Design review of the part built by this model. Coordinates are the model's own, in mm. A direction names the side the tool comes from. Round coordinates to 2 decimals unless told otherwise and drop trailing zeros. Order: outer loops, then holes, each group sorted by start corner. A loop starts at its lowest first (then second) coordinate and runs counter-clockwise, first axis right, second up. Notation, with made-up numbers: M -13,41 L 21,41 A19 cw 21,72 Z; hole C -15.75,85.25 d11. An arc over 180 degrees is marked long. Write each question's results on one line, items separated by ' | '. Start each with the question number.
Item 1: Wall thickness on line 1 (Y direction, x = 37, z = -0.35); line 2 (X direction, y = -19.05, z = -9); line 3 (Y direction, x = 8, z = -10.75): over which ranges is each line inside the solid? List them lowest first. Write a range as [from, to].
Item 2: Machinability: for faces 1 (the flat face through (-28, 0, -2)), 2 (the flat face through (12, 20, -11)), 3 (the cylindrical face through (-9.93, -20.09, -9.88)), which of the approach directions +Z, -Z, +X, -X, +Y, -Y give a long, thin tool a straight path to every point of the face, cutting with its end or side? Answer none if there is none.
Item 3: Take a section at A-A, the plane y = 0. Write out the cut boundary in (x, z), plus the area to 3 significant figures.
Item 4: Take a section at B-B, the plane x = 0. Write out the cut boundary in (y, z).
Item 5: Take a section at D-D, the plane z = -9. Write out the cut boundary in (x, y).
Item 6: Clearance check with flat-ended pins moving along their axes: pin 1 (9.5 mm diameter, centred on x = 40, y = 17.5, fed in from -Z); pin 2 (5 mm diameter, centred on y = -20.5, z = -14, fed in from +X); pin 3 (18 mm diameter, centred on x = -37, y = 0, fed in from +Z); pin 4 (1.5 mm diameter, centred on x = -25, z = -5.5, fed in from -Y). State where each tip first meets the part, or that it passes through.
Item 7: Take a section at C-C, the plane z = -5. Write out the cut boundary in (x, y).
Item 8: The part is to be moulded in two halves that separate along Y. For faces 4 (the flat face through (0, 15.75, -15)), 5 (the flat face through (-45, 0, -1)), 6 (the cylindrical face through (42.766, -16.629, -0.986)), 7 (the flat face through (-1, 22.5, -7)), say which applies: +Y half, -Y half, draft (parallel to the pull), parting line (faces both ways), or undercut.
```python
from build123d import *

# Parameters (mm, degrees)
SKETCH_1_W          = 90
SKETCH_1_H          = 45
SKETCH_1_R          = 2.9
SKETCH_1_R_2        = 7
EXTRUDE_2_DEPTH     = 2
EXTRUDE_3_DEPTH     = 2
SKETCH_3_R          = 15
CUT_EXTRUDE_1_DEPTH = 5
CUT_EXTRUDE_2_DEPTH = 1
EXTRUDE_4_DEPTH     = 13.5
SKETCH_5_R          = 1.3
CUT_EXTRUDE_3_DEPTH = 5.75
SKETCH_4_4_W        = 24.441241248
SKETCH_4_4_H        = 4.75
EXTRUDE_5_DEPTH     = 13.5
SKETCH_6_W          = 24.441241248
SKETCH_6_H          = 4
EXTRUDE_6_DEPTH     = 2


with BuildPart() as part:
    # Sketch 1 → Extrude 2 (new body)
    with BuildSketch(Plane.XY):
        Rectangle(SKETCH_1_W, SKETCH_1_H)
        with Locations((-40, 17.5)):
            Circle(SKETCH_1_R, mode=Mode.SUBTRACT)
        with Locations((-40, -17.5)):
            Circle(SKETCH_1_R, mode=Mode.SUBTRACT)
        with Locations((40, 17.5)):
            Circle(SKETCH_1_R, mode=Mode.SUBTRACT)
        with Locations((40, -17.5)):
            Circle(SKETCH_1_R, mode=Mode.SUBTRACT)
        with Locations((-37, 0)):
            Circle(SKETCH_1_R_2, mode=Mode.SUBTRACT)
        with Locations((37, 0)):
            Circle(SKETCH_1_R_2, mode=Mode.SUBTRACT)
    extrude(amount=-EXTRUDE_2_DEPTH)

    # Sketch 2 → Extrude 3 (add)
    with BuildSketch(Plane(origin=(0, 0, -2), x_dir=(-1, 0, 0), z_dir=(0, 0, -1))):
        Polygon((0, -22.5), (-25, -22.5), (-25, 22.5), (25, 22.5), (25, -22.5), align=None)
    extrude(amount=EXTRUDE_3_DEPTH)

    # Sketch 3 → Cut-Extrude 1 (cut, through all)
    with BuildSketch(Plane(origin=(0, 0, -4), x_dir=(-1, 0, 0), z_dir=(0, 0, -1))):
        Circle(SKETCH_3_R)
    extrude(amount=-CUT_EXTRUDE_1_DEPTH, mode=Mode.SUBTRACT)

    # Sketch 4 → Cut-Extrude 2 (cut)
    with BuildSketch(Plane(origin=(0, 0, -4), x_dir=(-1, 0, 0), z_dir=(0, 0, -1))):
        with BuildLine():
            Line((10.461237976, -10.75), (12.441241248, -10.75))
            Line((12.441241248, -10.75), (12.441241248, -8.379469924))
            ThreePointArc((12.441241248, -8.379469924), (11.512416856, -9.61583372), (10.461237976, -10.75))
        make_face()
        with BuildLine():
            Line((-12, -9), (-12, -10.75))
            Line((-12, -10.75), (-10.461237976, -10.75))
            ThreePointArc((-10.461237976, -10.75), (-11.264653917, -9.90492666), (-12, -9))
        make_face()
        with BuildLine():
            Line((-12, 2.25), (-12, -9))
            ThreePointArc((-12, -9), (-11.264653917, -9.90492666), (-10.461237976, -10.75))
            Line((-10.461237976, -10.75), (10.461237976, -10.75))
            ThreePointArc((10.461237976, -10.75), (11.512416856, -9.61583372), (12.441241248, -8.379469924))
            Line((12.441241248, -8.379469924), (12.441241248, 2.25))
            Line((12.441241248, 2.25), (-12, 2.25))
        make_face()
    extrude(amount=-CUT_EXTRUDE_2_DEPTH, mode=Mode.SUBTRACT)

    # Sketch 4_3 → Extrude 4 (add)
    with BuildSketch(Plane(origin=(0, 0, -4), x_dir=(-1, 0, 0), z_dir=(0, 0, -1))):
        Polygon((-12, -22.5), (0, -22.5), (12.441241248, -22.5), (12.441241248, -17.75), (-12, -17.75), align=None)
    extrude(amount=EXTRUDE_4_DEPTH)

    # Sketch 5 → Cut-Extrude 3 (cut, through all)
    with BuildSketch(Plane(origin=(0, -17.75, 0), x_dir=(1, 0, 0), z_dir=(0, 1, 0))):
        with Locations((-8.970620624, 9)):
            Circle(SKETCH_5_R)
        with Locations((8.529379376, 9)):
            Circle(SKETCH_5_R)
    extrude(amount=-CUT_EXTRUDE_3_DEPTH, mode=Mode.SUBTRACT)

    # Sketch 4_4 → Extrude 5 (add)
    with BuildSketch(Plane(origin=(0, 0, -4), x_dir=(-1, 0, 0), z_dir=(0, 0, -1))):
        with Locations((0.220620624, 20.125)):
            Rectangle(SKETCH_4_4_W, SKETCH_4_4_H)
    extrude(amount=EXTRUDE_5_DEPTH)

    # Sketch 6 → Extrude 6 (add)
    with BuildSketch(Plane.XZ.offset(-17.75)):
        with Locations((-0.220620624, -15.5)):
            Rectangle(SKETCH_6_W, SKETCH_6_H)
    extrude(amount=EXTRUDE_6_DEPTH)


solid = part.part
```
Results list:
1) line 1: [-22.5, -7], [7, 22.5] | line 2: [-12.44, -10.27], [-7.67, 7.23], [9.83, 12] | line 3: [-22.5, -17.75], [17.75, 22.5]
2) face 1: -Z, -X, +Y, -Y | face 2: -Z, +X, +Y, -Y | face 3: -Y
3) outline: M -45,-2 L -44,-2 L -44,0 L -45,0 Z; M -30,-2 L -25,-2 L -25,-4 L -15,-4 L -15,0 L -30,0 Z; M 15,-4 L 25,-4 L 25,-2 L 30,-2 L 30,0 L 15,0 Z; M 44,-2 L 45,-2 L 45,0 L 44,0 Z | area: 104 mm²
4) outline: M -22.5,-17.5 L -17.75,-17.5 L -17.75,-4 L -15,-4 L -15,0 L -22.5,0 Z; M 15,-4 L 17.75,-4 L 17.75,-13.5 L 15.75,-13.5 L 15.75,-17.5 L 22.5,-17.5 L 22.5,0 L 15,0 Z
5) outline: M -12.44,-22.5 L -10.27,-22.5 L -10.27,-17.75 L -12.44,-17.75 Z; M -12.44,17.75 L 12,17.75 L 12,22.5 L -12.44,22.5 Z; M -7.67,-22.5 L 7.23,-22.5 L 7.23,-17.75 L -7.67,-17.75 Z; M 9.83,-22.5 L 12,-22.5 L 12,-17.75 L 9.83,-17.75 Z
6) pin 1: z = -2 | pin 2: x = 12 | pin 3: z = 0 | pin 4: through
7) outline: M -12.44,-22.5 L 12,-22.5 L 12,-17.75 L -12.44,-17.75 Z; M -12.44,17.75 L 12,17.75 L 12,22.5 L -12.44,22.5 Z
8) face 4: undercut | face 5: draft | face 6: undercut | face 7: +Y half
